For this review, take the finished solid that the model builds, in its own axes (mm). A direction names the side the tool comes from. Give positions to 0.01 mm unless a question says otherwise; leave off trailing zeros. Loops run counter-clockwise (first coordinate to the right, second up) from the corner with the lowest first, then second, coordinate; pieces in that order, holes last. Notation, with made-up numbers: (52, 66.5) -> (81, 66.5) arc R20 ccw to (81, 81.5) -> close; hole circle Ø9 at (74.5, 0.5). An arc over 180 degrees is marked (long way). One line per question, with ' | ' between items. Start each with the question number.
(1) Consider section C-C (y = -19). Write out the cut boundary in (x, z), and give its area (3 significant figures).
(2) Consider section B-B (x = -12.5). Write out the cut boundary in (y, z).
(3) Wall thickness on probe 1 along Z at (x, y) = (-4.5, -10); probe 2 along Z at (x, y) = (-63, -14); probe 3 along X at (y, z) = (10, -15.5): over which ranges is each line inside the solid? List them lowest first.
(4) Consider section A-A (z = 39.5). Write out the cut boundary in (x, y), and give its area (3 significant figures).
(5) Tool access review of faces 1 (the cylindrical face through (-0.1, -0.35, 44.38)), 2 (the cylindrical face through (2.41, -0.35, 46.38)): name each direction out of +Z, -Z, +X, -X, +Y, -Y from which nothing blocks a thin tool from reaching the whole face with its end or side.
(6) Insertion check: P1, Ø8, axis at x = -45.5, y = -11, coming from the -Z side; P2, Ø12, axis at x = 33, y = -9, coming from the -Z side; P3, Ø4, axis at x = -52, y = 11.5, coming from the -Z side. Each pin has a flat end and moves straight along its axis. Give the tip position at first contact, or say it passes through.
from build123d import *

# Parameters (mm, degrees)
F1_DEPTH = 25


with BuildPart() as f1:
    # F0 (on Front) → F1 (new body, symmetric)
    with BuildSketch(Plane.XZ):
        with BuildLine():
            ThreePointArc((74.354294, -0.612335), (74.558297, -0.10376), (74.463656, 0.435969))
            ThreePointArc((74.463656, 0.435969), (1.137581, 46.391442), (-72.188495, 0.435969))
            ThreePointArc((-72.188495, 0.435969), (-72.283136, -0.10376), (-72.079132, -0.612335))
            ThreePointArc((-72.079132, -0.612335), (1.137581, -36.513716), (74.354294, -0.612335))
        make_face()
        with BuildLine():
            ThreePointArc((-70.115532, 0.12209), (1.137581, 44.391442), (72.390694, 0.12209))
            ThreePointArc((72.390694, 0.12209), (1.137581, -34.513716), (-70.115532, 0.12209))
        make_face(mode=Mode.SUBTRACT)
    extrude(amount=F1_DEPTH, both=True)


solid = f1.part
A:
1) outline: (-72.19, 0.44) arc R1 ccw to (-72.08, -0.61) arc R92.61 ccw to (74.35, -0.61) arc R1 ccw to (74.46, 0.44) arc R81.48 ccw to start; hole (-70.12, 0.12) arc R90.61 ccw to (72.39, 0.12) arc R79.48 ccw to start | area: 694 mm^2
2) outline: (-25, -35.5) -> (25, -35.5) -> (25, -33.48) -> (-25, -33.48) -> close; (-25, 43.21) -> (25, 43.21) -> (25, 45.24) -> (-25, 45.24) -> close
3) probe 1: z = -36.34 to -34.34, 44.19 to 46.2 | probe 2: z = -10.71 to -7.91, 11.85 to 15.16 | probe 3: x = -57.6 to -54.4, 56.67 to 59.88
4) outline: (-31.66, -25) -> (-26.31, -25) -> (-26.31, 25) -> (-31.66, 25) -> close; (28.59, -25) -> (33.93, -25) -> (33.93, 25) -> (28.59, 25) -> close | area: 534 mm^2
5) face 1: +Y, -Y | face 2: +Z, +Y, -Y
6) P1: stops at z = -26.11 | P2: stops at z = -32.83 | P3: stops at z = -21.11
